CAD build for the part. Positions are in the model's coordinates, mm. Face numbers are marked on the shaded views. A direction names the side the tool comes from. Give positions to 0.01 mm unless a question says otherwise; leave off trailing zeros. Loops run counter-clockwise (first coordinate to the right, second up) from the corner with the lowest first, then second, coordinate; pieces in that order, holes last. Notation, with made-up numbers: (-40, 38.25) -> (2, 38.25) arc R19 ccw to (2, 74.25) -> close; hole circle Ø3 at (-21.75, 67.5). An arc over 180 degrees is marked (long way). Use one line per item in the form item = value.
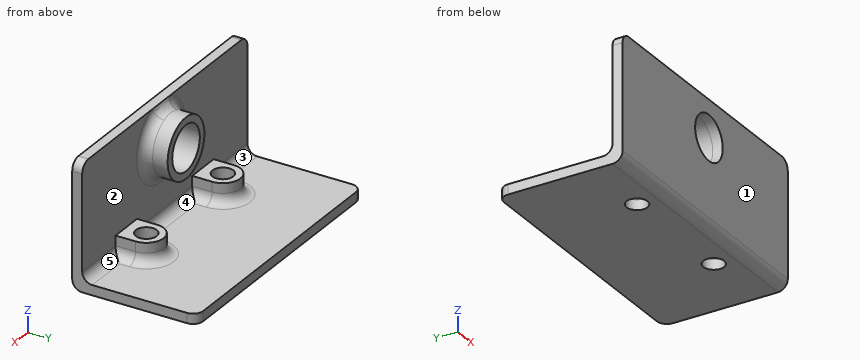
```python
from build123d import *

# Parameters (mm, degrees)
SKETCH1_W           = 53.9
SKETCH1_H           = 25
BOSS_EXTRUDE1_DEPTH = 2
SKETCH2_W           = 53.9
SKETCH2_H           = 2
BOSS_EXTRUDE2_DEPTH = 23
SKETCH3_R           = 2.1
CUT_EXTRUDE1_DEPTH  = 3
SKETCH4_R           = 4.5
CUT_EXTRUDE2_DEPTH  = 3
SKETCH5_R           = 2.1
BOSS_EXTRUDE3_DEPTH = 4
SKETCH6_R           = 6
SKETCH6_R_2         = 4.5
BOSS_EXTRUDE4_DEPTH = 5
FILLET1_R           = 2


with BuildPart() as part:
    # Sketch1 → Boss-Extrude1 (new body)
    with BuildSketch(Plane.XY):
        with Locations((26.95, 12.5)):
            Rectangle(SKETCH1_W, SKETCH1_H)
    extrude(amount=BOSS_EXTRUDE1_DEPTH)

    # Sketch2 → Boss-Extrude2 (add)
    with BuildSketch(Plane.XY.offset(2)):
        with Locations((26.95, 1)):
            Rectangle(SKETCH2_W, SKETCH2_H)
    extrude(amount=BOSS_EXTRUDE2_DEPTH)

    # Sketch3 → Cut-Extrude1 (cut, through all)
    with BuildSketch(Plane.XY.offset(2)):
        with Locations((39.5, 6)):
            Circle(SKETCH3_R)
        with Locations((14.5, 6)):
            Circle(SKETCH3_R)
    extrude(amount=-CUT_EXTRUDE1_DEPTH, mode=Mode.SUBTRACT)

    # Sketch4 → Cut-Extrude2 (cut, through all)
    with BuildSketch(Plane(origin=(0, 2, 0), x_dir=(1, 0, 0), z_dir=(0, 1, 0))):
        with Locations((28.167949192, -17.557050808)):
            Circle(SKETCH4_R)
    extrude(amount=-CUT_EXTRUDE2_DEPTH, mode=Mode.SUBTRACT)

    # Sketch5 → Boss-Extrude3 (add)
    with BuildSketch(Plane.XY.offset(2)):
        with BuildLine():
            Line((18, 6), (18, 2))
            Line((18, 2), (11, 2))
            Line((11, 2), (11, 6))
            ThreePointArc((11, 6), (14.5, 9.5), (18, 6))
        make_face()
        with Locations((14.5, 6)):
            Circle(SKETCH5_R, mode=Mode.SUBTRACT)
        with BuildLine():
            Line((36, 6), (36, 2))
            Line((36, 2), (43, 2))
            Line((43, 2), (43, 6))
            ThreePointArc((43, 6), (39.5, 9.5), (36, 6))
        make_face()
        with Locations((39.5, 6)):
            Circle(SKETCH5_R, mode=Mode.SUBTRACT)
    extrude(amount=BOSS_EXTRUDE3_DEPTH)

    # Sketch6 → Boss-Extrude4 (add)
    with BuildSketch(Plane(origin=(0, 2, 0), x_dir=(1, 0, 0), z_dir=(0, 1, 0))):
        with Locations((28.167949192, -17.557050808)):
            Circle(SKETCH6_R)
        with Locations((28.167949192, -17.557050808)):
            Circle(SKETCH6_R_2, mode=Mode.SUBTRACT)
    extrude(amount=BOSS_EXTRUDE4_DEPTH)

    # Fillet1
    fillet1_edges = [part.edges().sort_by_distance(p)[0] for p in [
        (48.45, 2, 2),
        (0, 1, 25),
        (53.9, 1, 25),
        (5.5, 2, 2),
        (14.5, 9.5, 2),
        (11, 4, 2),
        (18, 4, 2),
        (27, 2, 2),
        (26.95, 0, 0),
        (39.5, 9.5, 2),
        (36, 4, 2),
        (43, 4, 2),
        (22.167949192, 2, 17.557050808),
        (0, 25, 1),
        (53.9, 25, 1),
    ]]
    fillet(fillet1_edges, radius=FILLET1_R)


solid = part.part
```
1. Cut at C-C, the plane y = 18. Write the cut outline in (x, z).
Result sheet:
outline = (0, 0) -> (53.9, 0) -> (53.9, 2) -> (0, 2) -> close
2. Drill centre lines: line 1 (X direction, y = 6.75, z = 3.75); line 2 (X direction, y = 4.5, z = 1.5); line 3 (X direction, y = 7.75, z = 4.25). Where is each one in solid material? Low to high.
Result sheet:
line_1 = 11.07 to 12.54, 16.46 to 17.93, 36.07 to 37.54, 41.46 to 42.93
line_2 = 0 to 13.03, 15.97 to 38.03, 40.97 to 53.9
line_3 = 11.47 to 13.34, 15.66 to 17.53, 36.47 to 38.34, 40.66 to 42.53
3. Tool access for the marked faces 1, 2 and 3: list every direction of +Z, -Z, +X, -X, +Y, -Y with a clear straight run to the whole face (end or side of a thin tool).
Result sheet:
face_1 = +Z, -Z, +X, -X, -Y
face_2 = +Y
face_3 = +Z, -X, +Y
4. Drop flat-ended pins along their axis: P1, Ø3.5, axis at x = 41, y = 6, coming from the +Z side; P2, Ø3, axis at x = 32.5, y = 7, coming from the +Z side; P3, Ø1.5, axis at x = 12.5, z = 6.5, coming from the +Y side. Give the stop position or say it passes through.
Result sheet:
P1 = 6
P2 = 22.85
P3 = 9.19
5. Mould opens along X. For the marked faces 4 and 5 say: pulls with the +X half, pulls with the -X half, needs draft (parallel to the pull), parting line crosses it, or undercut.
Result sheet:
face_4 = undercut
face_5 = needs draft
6. Cut at B-B, the plane y = 3. State how many separate pieces and enclosed holes the cut face has, then the cut area to 3 significant figures.
Result sheet:
separate_pieces = 2
enclosed_holes = 1
area = 236 mm^2
7. Cut at A-A, the plane x = 14.5. Write the cut outline in (y, z).
Result sheet:
outline = (0, 2) arc R2 ccw to (2, 0) -> (3.9, 0) -> (3.9, 6) -> (2, 6) -> (2, 25) -> (0, 25) -> close; (8.1, 0) -> (25, 0) -> (25, 2) -> (11.5, 2) arc R2 cw to (9.5, 4) -> (9.5, 6) -> (8.1, 6) -> close
